Could you check a few things on this model? Use its own coordinates, in mm. A direction names the side the tool comes from. Round coordinates to 2 decimals unless told otherwise and drop trailing zeros. Loops run counter-clockwise (first coordinate to the right, second up) from the corner with the lowest first, then second, coordinate; pieces in that order, holes last. Notation, with made-up numbers: M 16.25,24.25 L 45.25,24.25 A28 ccw 45.25,56.25 Z; hole C 23,44.25 d6. An arc over 180 degrees is marked long. One line per item, written item: value. Start each with the question number.
Q1. Which directions (+Z, -Z, +X, -X, +Y, -Y) give clear straight access to the entire face, cutting with the end or side of a thin tool? Please do faces 5 (the face through (5, -10, 1)), 6 (the face through (10, -81, 2)), 7 (the face through (5, -149, 1)), 8 (the face through (6.75, -151.26, 4.51)).
Q2. Imagine slicing it at B-B (x = 5). Please give me the cut outline in (y, z), then the cut area to 3 significant figures.
Q3. Please list where these lines run through material, in increasing order: line 1 along Y through (x, z) = (5, 1.85); line 2 along Y through (x, z) = (5, 4.2); line 3 along Z through (x, y) = (3, -151.5).
Q4. Thinking about a two-plate mould opening in Y: for faces 1 (the face through (4.239, -155.464, 2.479)), 2 (the face through (5, -78, 5)), 3 (the face through (6.4, -155.4, 4)), 4 (the face through (5, 0, 3)), which applies, released by +Y, released by -Y, zero draft, split by the parting line, or undercut?
Q5. Imagine slicing it at A-A (y = -154). Please give me the cut outline in (x, z), then the cut area to 3 significant figures.
Q6. I'm going to push flat-ended pins straight in: pin 1 Ø5 at (x, y) = (4, -6) entering from -Z; pin 2 Ø6 at (x, y) = (5, -154) entering from +Z; pin 3 Ø0.5 at (x, z) = (5, 0.5) entering from -Y. Where does each tip first touch, or does it pass through?
Q7. Imagine slicing it at C-C (y = -14). Please give me the cut outline in (x, z), then the cut area to 3 significant figures.
from build123d import *

# Parameters (mm, degrees)
SKETCH_1_W          = 10
SKETCH_1_H          = 159
EXTRUDE_1_DEPTH     = 5
SKETCH_3_W          = 10
SKETCH_3_H          = 20
CUT_EXTRUDE_1_DEPTH = 1
HOLE_WIZARD_M4_1_D  = 3.3
SKETCH_7_R          = 3.25
CUT_EXTRUDE_2_DEPTH = 1


with BuildPart() as part:
    # 草图1 → 凸台-拉伸1 (new body)
    with BuildSketch(Plane.XY):
        with Locations((5, -79.5)):
            Rectangle(SKETCH_1_W, SKETCH_1_H)
    extrude(amount=EXTRUDE_1_DEPTH)

    # 草图3 → 切除-拉伸1 (cut)
    with BuildSketch(Plane(origin=(0, 0, 0), x_dir=(-1, 0, 0), z_dir=(0, 0, -1))):
        with Locations((-5, -10)):
            Rectangle(SKETCH_3_W, SKETCH_3_H)
        with Locations((-5, -149)):
            Rectangle(SKETCH_3_W, SKETCH_3_H)
    extrude(amount=-CUT_EXTRUDE_1_DEPTH, mode=Mode.SUBTRACT)

    # M4 螺纹孔的螺纹孔钻头1 (through all)
    with Locations(Plane.XY.offset(5)):
        with Locations((5, -5), (5, -154)):
            Hole(HOLE_WIZARD_M4_1_D / 2)

    # 草图7 → 切除-拉伸2 (cut)
    with BuildSketch(Plane.XY.offset(5)):
        with Locations((5, -5)):
            Circle(SKETCH_7_R)
        with Locations((5, -154)):
            Circle(SKETCH_7_R)
    extrude(amount=-CUT_EXTRUDE_2_DEPTH, mode=Mode.SUBTRACT)


solid = part.part
Report:
1. face 5: -Z, +X, -X, +Y
1. face 6: +Z, -Z, +X, +Y, -Y
1. face 7: -Z, +X, -X, -Y
1. face 8: +Z
2. outline: M -159,1 L -155.65,1 L -155.65,4 L -157.25,4 L -157.25,5 L -159,5 Z; M -152.35,1 L -139,1 L -139,0 L -20,0 L -20,1 L -6.65,1 L -6.65,4 L -8.25,4 L -8.25,5 L -150.75,5 L -150.75,4 L -152.35,4 Z; M -3.35,1 L 0,1 L 0,5 L -1.75,5 L -1.75,4 L -3.35,4 Z
2. area: 722 mm²
3. line 1: y = -159 to -155.65, -152.35 to -6.65, -3.35 to 0
3. line 2: y = -159 to -157.25, -150.75 to -8.25, -1.75 to 0
3. line 3: z = 1 to 4
4. face 1: undercut
4. face 2: zero draft
4. face 3: undercut
4. face 4: released by +Y
5. outline: M 0,1 L 3.35,1 L 3.35,4 L 1.75,4 L 1.75,5 L 0,5 Z; M 6.65,1 L 10,1 L 10,5 L 8.25,5 L 8.25,4 L 6.65,4 Z
5. area: 23.6 mm²
6. pin 1: stops at z = 1
6. pin 2: stops at z = 4
6. pin 3: stops at y = -139
7. outline: M 0,1 L 10,1 L 10,5 L 0,5 Z
7. area: 40.0 mm²
